from build123d import *

# Parameters (mm, degrees)
BOSS_EXTRUDE1_DEPTH      = 254.000001
BOSS_EXTRUDE1_DEPTH_BACK = 254.000001
SKETCH3_W                = 50.8
SKETCH3_H                = 25.4
SKETCH3_W_2              = 47.625
SKETCH3_H_2              = 22.225
F_10_CLEARANCE_HOLE1_D   = 4.9784
F_10_CLEARANCE_HOLE2_D   = 4.9784
SKETCH11_R               = 9.525
CUT_EXTRUDE1_DEPTH       = 257.527426425


with BuildPart() as part:
    # Sketch3 → Boss-Extrude1 (new, two sides: drawn at the far end of the back side and taken through both)
    with BuildSketch(Plane.XY.offset(-BOSS_EXTRUDE1_DEPTH_BACK)):
        Rectangle(SKETCH3_W, SKETCH3_H)
        Rectangle(SKETCH3_W_2, SKETCH3_H_2, mode=Mode.SUBTRACT)
    extrude(amount=BOSS_EXTRUDE1_DEPTH + BOSS_EXTRUDE1_DEPTH_BACK)

    # #10 Clearance Hole1 (through all)
    with Locations(Plane(origin=(25.4, 0, 0), x_dir=(0, 0, -1), z_dir=(1, 0, 0))):
        with Locations((-241.300000508, 0), (-215.900000508, 0), (215.899999492, 0), (241.299999492, 0)):
            Hole(F_10_CLEARANCE_HOLE1_D / 2)

    # #10 Clearance Hole2 (through all)
    with Locations(Plane(origin=(0, 12.7, 0), x_dir=(1, 0, 0), z_dir=(0, 1, 0))):
        with Locations((-13.207999909, -179.867533038), (12.192000091, -179.867533038), (-15.875, -234.950000508), (15.875, -234.950000508)):
            Hole(F_10_CLEARANCE_HOLE2_D / 2)

    # Sketch11 → Cut-Extrude1 (cut, through all)
    with BuildSketch(Plane(origin=(0, 12.7, 0), x_dir=(1, 0, 0), z_dir=(0, 1, 0))):
        with Locations(Location((0, 228.600000508, 0), (0, 0, 180))):
            Circle(SKETCH11_R)
    extrude(amount=-CUT_EXTRUDE1_DEPTH, mode=Mode.SUBTRACT)


solid = part.part
Could you check a few things on this model? Use its own coordinates, in mm. A direction names the side the tool comes from. Give positions to 0.01 mm unless a question says otherwise; leave off trailing zeros. Order: outer loops, then holes, each group sorted by start corner. A loop starts at its lowest first (then second) coordinate and runs counter-clockwise, first axis right, second up.
1. We'd pull the mould along X, two halves only. Please class faces 1 (the flat face through (-25.4, 0, -4)), 2 (the flat face through (0, -11.112, -4)), 3 (the flat face through (0, -12.7, -4)), 4 (the flat face through (23.812, 0, -4)): pulls with the +X half, pulls with the -X half, needs draft (parallel to the pull), parting line crosses it, or undercut.
2. Suppose I cut it at C-C (z = -228.6). List the corners of the cut face in (x, y) for me (1 decimal), plus the area to 3 significant figures.
3. Will these pins go through, and if not, where does the flat tip stop? P1, Ø4, axis at x = 12.19, z = 179.87, coming from the -Y side; P2, Ø8, axis at y = 0, z = -241.3, coming from the +X side.
4. Suppose I cut it at A-A (z = 139.5). List the corners of the cut face in (x, y) for me, plus the area to 3 significant figures.
5. Suppose I cut it at B-B (x = 0). List the corners of the cut face in (y, z) for me (1 decimal).
6. I need wall thicknesses on L1, parallel to X at y = 10, z = 117; L2, parallel to Z at x = -0.5, y = 11.75; L3, parallel to X at y = 11.95, z = -228.6 (3 decimals). Which ranges of each line are inside material? Lowest first, please.
7. For faces 5 (the flat face through (0, 12.7, -4)), 6 (the flat face through (0, 11.112, -4)), which set-ups out of +Z, -Z, +X, -X, +Y, -Y let a thin tool reach every point of the face, with its end or its side?
Solved:
1. face 1: pulls with the -X half
1. face 2: undercut
1. face 3: needs draft
1. face 4: undercut
2. outline: (-25.4, -12.7) - (-9.5, -12.7) - (-9.5, -11.1) - (-23.8, -11.1) - (-23.8, 11.1) - (-9.5, 11.1) - (-9.5, 12.7) - (-25.4, 12.7) - close; (9.5, -12.7) - (25.4, -12.7) - (25.4, 12.7) - (9.5, 12.7) - (9.5, 11.1) - (23.8, 11.1) - (23.8, -11.1) - (9.5, -11.1) - close
2. area: 171 mm2
3. P1: passes through
3. P2: stops at x = 25.4
4. outline: (-25.4, -12.7) - (25.4, -12.7) - (25.4, 12.7) - (-25.4, 12.7) - close; hole (-23.81, -11.11) - (23.81, -11.11) - (23.81, 11.11) - (-23.81, 11.11) - close
4. area: 232 mm2
5. outline: (-12.7, -254) - (-11.1, -254) - (-11.1, -238.1) - (-12.7, -238.1) - close; (-12.7, -219.1) - (-11.1, -219.1) - (-11.1, 254) - (-12.7, 254) - close; (11.1, -254) - (12.7, -254) - (12.7, -238.1) - (11.1, -238.1) - close; (11.1, -219.1) - (12.7, -219.1) - (12.7, 254) - (11.1, 254) - close
6. L1: x = -25.4 to -23.81, 23.81 to 25.4
6. L2: z = -254 to -238.11, -219.09 to 254
6. L3: x = -25.4 to -9.525, 9.525 to 25.4
7. face 5: +Z, -Z, +X, -X, +Y
7. face 6: +Z, -Z
